For this review, take the finished solid that the model builds, in its own axes (mm). Give positions to 0.01 mm unless a question says otherwise; leave off trailing zeros. Loops run counter-clockwise (first coordinate to the right, second up) from the corner with the lowest first, then second, coordinate; pieces in that order, holes last. Notation, with made-up numbers: M 17.5,39 L 48.5,39 A16 cw 48.5,54 Z; hole C 61,-20 d9. An arc over 180 degrees is marked long. Use CSV: the item, a comma, the result in double quotes. Start each with the question number.
1. Take a section at A-A, the plane x = -48.75. Write out the cut boundary in (y, z).
2. Take a section at C-C, the plane y = 2. State how many separate pieces and enclosed holes the cut face has, and give its area (3 significant figures).
3. Insertion check: P1, Ø5, axis at x = 48.75, z = -10, coming from the -Y side; P2, Ø5.5, axis at x = -48.75, z = -140, coming from the -Y side; P3, Ø1.5, axis at x = -2.5, y = -1.5, coming from the -Z side; P4, Ø5, axis at x = -48.75, z = -10, coming from the +Y side. Each pin has a flat end and moves straight along its axis. Give the tip position at first contact, or say it passes through.
4. Take a section at D-D, the plane z = -140. Write out the cut boundary in (x, y).
5. To check wall thickness, follow line 1 (X direction, y = 1.45, z = -30); line 2 (X direction, y = 2, z = -78.5) (3 decimals); line 3 (X direction, y = 0.15, z = -140). State the ranges of each line that lie inside material, in increasing order. Write a range as [from, to].
6. Take a section at B-B, the plane z = -30. Write out the cut boundary in (x, y).
from build123d import *

# Parameters (mm, degrees)
SKETCH_1_R          = 2.1
EXTRUDE_1_DEPTH     = 3
SKETCH_2_R          = 1
CUT_EXTRUDE_1_DEPTH = 166.113786523
CHAMFER_1_SIZE      = 4
CHAMFER_2_SIZE      = 2


with BuildPart() as part:
    # 草图1 → 凸台-拉伸1 (new, symmetric)
    with BuildSketch(Plane(origin=(0, 0, 0), x_dir=(1, 0, 0), z_dir=(0, 1, 0))):
        Polygon((-68.75, 150), (-68.75, 50), (-58.75, 50), (-58.75, 0), (58.75, 0), (58.75, 40), (-38.75, 150), align=None)
        with Locations(Location((-48.75, 140, 0), (0, 0, 270))):
            Circle(SKETCH_1_R, mode=Mode.SUBTRACT)
        with Locations(Location((-48.75, 10, 0), (0, 0, 270))):
            Circle(SKETCH_1_R, mode=Mode.SUBTRACT)
        with Locations(Location((-28.75, 30, 0), (0, 0, 270))):
            Circle(SKETCH_1_R, mode=Mode.SUBTRACT)
        with Locations(Location((28.75, 30, 0), (0, 0, 270))):
            Circle(SKETCH_1_R, mode=Mode.SUBTRACT)
        with Locations(Location((-28.75, 10, 0), (0, 0, 270))):
            Circle(SKETCH_1_R, mode=Mode.SUBTRACT)
        with Locations(Location((28.75, 10, 0), (0, 0, 270))):
            Circle(SKETCH_1_R, mode=Mode.SUBTRACT)
        with Locations(Location((48.75, 30, 0), (0, 0, 270))):
            Circle(SKETCH_1_R, mode=Mode.SUBTRACT)
        with Locations(Location((48.75, 10, 0), (0, 0, 270))):
            Circle(SKETCH_1_R, mode=Mode.SUBTRACT)
    extrude(amount=EXTRUDE_1_DEPTH, both=True)

    # 草图2 → 切除-拉伸1 (cut, through all)
    with BuildSketch(Plane(origin=(0, 3, 0), x_dir=(1, 0, 0), z_dir=(0, 1, 0))):
        with Locations((-58.75, 49)):
            Circle(SKETCH_2_R)
    extrude(amount=-CUT_EXTRUDE_1_DEPTH, mode=Mode.SUBTRACT)

    # 倒角1
    chamfer_1_edges = [part.edges().sort_by_distance(p)[0] for p in [
        (58.75, 0, 0),
        (-58.75, 0, 0),
        (-68.75, 0, -50),
        (-68.75, 0, -150),
    ]]
    chamfer(chamfer_1_edges, length=CHAMFER_1_SIZE)

    # 倒角2
    chamfer_2_edges = [part.edges().sort_by_distance(p)[0] for p in [
        (-48.75, -3, -142.1),
        (-28.75, -3, -32.1),
        (-48.75, -3, -12.1),
        (28.75, -3, -32.1),
        (-28.75, -3, -12.1),
        (28.75, -3, -12.1),
        (48.75, -3, -12.1),
        (48.75, -3, -32.1),
    ]]
    chamfer(chamfer_2_edges, length=CHAMFER_2_SIZE)


solid = part.part
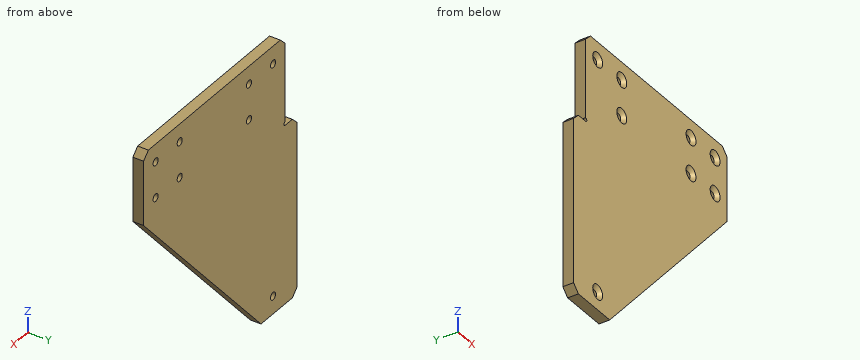
Result set:
1,outline,"M -3,-150 L 3,-150 L 3,-142.1 L -1,-142.1 L -3,-144.1 Z; M -3,-135.9 L -1,-137.9 L 3,-137.9 L 3,-12.1 L -1,-12.1 L -3,-14.1 Z; M -3,-5.9 L -1,-7.9 L 3,-7.9 L 3,0 L -3,0 Z"
2,separate pieces,"1"
2,enclosed holes,"8"
2,area,"13,100 mm2"
3,P1,"y = -1.4"
3,P2,"y = -1.65"
3,P3,"z = -109.95"
3,P4,"y = 3"
4,outline,"M -68.75,-3 L -52.85,-3 L -50.85,-1 L -50.85,3 L -68.75,3 Z; M -46.65,-1 L -44.65,-3 L -29.89,-3 L -29.89,3 L -46.65,3 Z"
5,line 1,"[-58.75, -30.85], [-26.65, 26.65], [30.85, 46.65], [50.85, 58.75]"
5,line 2,"[-68.75, 24.625]"
5,line 3,"[-68.75, -50.85], [-46.65, -29.89]"
6,outline,"M -58.75,-3 L -32.85,-3 L -30.85,-1 L -30.85,3 L -58.75,3 Z; M -26.65,-1 L -24.65,-3 L 24.65,-3 L 26.65,-1 L 26.65,3 L -26.65,3 Z; M 30.85,-1 L 32.85,-3 L 44.65,-3 L 46.65,-1 L 46.65,3 L 30.85,3 Z; M 50.85,-1 L 52.85,-3 L 58.75,-3 L 58.75,3 L 50.85,3 Z"
